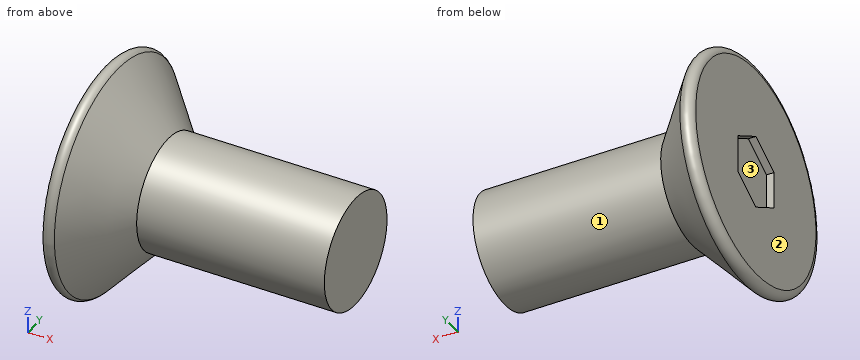
```python
from build123d import *

# Parameters (mm, degrees)
CONG_1_R                = 0.2
ENL_V_MAT_EXTRU_1_DEPTH = 0.2


with BuildPart() as part:
    # Esquisse1 → Révolution1 (revolve)
    with BuildSketch(Plane.XY, mode=Mode.PRIVATE) as r_volution1_sk:
        Polygon((0, 0), (0, 3.4), (1.7, 1.5), (6.7, 1.5), (6.7, 0), align=None)
    revolve(r_volution1_sk.sketch.rotate(Axis((0, 0, 0), (1, 0, 0)), 90), axis=Axis((0, 0, 0), (1, 0, 0)))

    # Congé1
    cong_1_edges = [part.edges().sort_by_distance(p)[0] for p in [
        (0, 0, -3.4),
    ]]
    fillet(cong_1_edges, radius=CONG_1_R)

    # Esquisse2 → Enlèv. mat.-Extru.1 (cut)
    with BuildSketch(Plane.ZY):
        Polygon((0.5, -0.866025404), (1, 0), (0.5, 0.866025404), (-0.5, 0.866025404), (-1, 0), (-0.5, -0.866025404), align=None)
    extrude(amount=-ENL_V_MAT_EXTRU_1_DEPTH, mode=Mode.SUBTRACT)


solid = part.part
```
Model file for the job. Use its own axes, mm. Face numbers are marked on the shaded views. Give positions to 0.01 mm unless a question says otherwise; leave off trailing zeros. Write each loop counter-clockwise with the first axis right and the second up, starting at its lowest first coordinate (ties: lowest second). Pieces come first, ordered by that corner, then holes. Notation, with made-up numbers: M 40.25,-33 L 87.25,-33 A21 cw 87.25,-7 Z; hole C 30,76 d6. An arc over 180 degrees is marked long. Use a Markdown table: item, result.
1) Cut at A-A (z = 0). List the corners of the cut face in (x, y), and give its area (3 significant figures).
Responses:
| item | result |
|---|---|
| outline | M 0,-2.88 A0.2 ccw 0.35,-3.01 L 1.7,-1.5 L 6.7,-1.5 L 6.7,1.5 L 1.7,1.5 L 0.35,3.01 A0.2 ccw 0,2.88 L 0,0.87 L 0.2,0.87 L 0.2,-0.87 L 0,-0.87 Z |
| area | 22.9 mm2 |
2) Pull direction Y, two halves, no side cores. Call the marked faces 1, 2 and 3: +Y half, -Y half, draft (parallel to the pull), parting line (faces both ways), or undercut.
Responses:
| item | result |
|---|---|
| face 1 | parting line |
| face 2 | draft |
| face 3 | undercut |
3) Cut at C-C (x = 1). List the corners of the cut face in (y, z), and give its area (3 significant figures).
Responses:
| item | result |
|---|---|
| outline | C 0,0 d4.56 |
| area | 16.4 mm2 |
4) Cut at B-B (x = 5.5). List the corners of the cut face in (y, z).
Responses:
| item | result |
|---|---|
| outline | C 0,0 d3 |
5) Drill centre lines: line 1 (X direction, y = -0.25, z = -0.75); line 2 (Y direction, x = 1, z = 1.75); line 3 (X direction, y = 2, z = -0.5). Where is each one in solid material? Low to high. Write a range as from..to.
Responses:
| item | result |
|---|---|
| line 1 | x = 0.2..6.7 |
| line 2 | y = -1.47..1.47 |
| line 3 | x = 0..1.2 |
6) Pin check, flat tips, straight feed: pin 1 (2 mm diameter, centred on x = 1, y = -1.5, fed in from +Z); pin 2 (3 mm diameter, centred on x = 2, y = 0, fed in from -Z); pin 3 (2 mm diameter, centred on x = 3.5, y = 1, fed in from +Z). Stop position of each tip, or through.
Responses:
| item | result |
|---|---|
| pin 1 | stops at z = 2.95 |
| pin 2 | stops at z = -2.84 |
| pin 3 | stops at z = 1.5 |
